Read the model definition and answer for the solid it produces. Units are mm, in the model's axes. A direction names the side the tool comes from. Coordinates: 2 decimals unless noted, no trailing zeros. Order: outer loops, then holes, each group sorted by start corner. A loop starts at its lowest first (then second) coordinate and runs counter-clockwise, first axis right, second up.
```python
from build123d import *

# Parameters (mm, degrees)
F1_DEPTH = 100
F2_R     = 8.25
F3_DEPTH = 130.001
F4_R     = 20


with BuildPart() as f1:
    # F0 (on Top) → F1 (new body, symmetric)
    with BuildSketch(Plane.XY):
        with BuildLine():
            Line((-45, -45), (45, -45))
            ThreePointArc((45, -45), (59.142136, -39.142136), (65, -25))
            Line((65, -25), (65, 45))
            Line((65, 45), (55, 45))
            Line((55, 45), (55, -25))
            ThreePointArc((55, -25), (52.071068, -32.071068), (45, -35))
            Line((45, -35), (-45, -35))
            ThreePointArc((-45, -35), (-52.071068, -32.071068), (-55, -25))
            Line((-55, -25), (-55, 45))
            Line((-55, 45), (-65, 45))
            Line((-65, 45), (-65, -25))
            ThreePointArc((-65, -25), (-59.142136, -39.142136), (-45, -45))
        make_face()
    extrude(amount=F1_DEPTH, both=True)

    # F2 (on face) → F3 (cut, through all)
    with BuildSketch(Plane.YZ.offset(65)):
        with Locations((0, 62.5)):
            Circle(F2_R)
        with Locations((0, -62.5)):
            Circle(F2_R)
    extrude(amount=-F3_DEPTH, mode=Mode.SUBTRACT)

    # F4
    f4_edges = [f1.edges().sort_by_distance(p)[0] for p in [
        (60, 45, 100),
        (-60, 45, 100),
        (-60, 45, -100),
        (60, 45, -100),
    ]]
    fillet(f4_edges, radius=F4_R)


solid = f1.part
```
1) Determine the mould class of faces 1 (the cylindrical face through (58.986, -39.297, 1.4)), 2 (the cylindrical face through (-59.93, -1.07, 70.68)), 3 (the flat face through (65, 10, 1)), 4 (the cylindrical face through (59.93, 38.986, -94.297)) for opening direction Y: pulls with the +Y half, pulls with the -Y half, needs draft (parallel to the pull), parting line crosses it, or undercut.
A:
face 1: pulls with the -Y half
face 2: undercut
face 3: needs draft
face 4: pulls with the +Y half
2) A cutting plane is placed at B-B, the plane y = 0. Determine the outline of the cut face in (x, z).
A:
outline: (-65, -100) - (-55, -100) - (-55, -70.75) - (-65, -70.75) - close; (-65, -54.25) - (-55, -54.25) - (-55, 54.25) - (-65, 54.25) - close; (-65, 70.75) - (-55, 70.75) - (-55, 100) - (-65, 100) - close; (55, -100) - (65, -100) - (65, -70.75) - (55, -70.75) - close; (55, -54.25) - (65, -54.25) - (65, 54.25) - (55, 54.25) - close; (55, 70.75) - (65, 70.75) - (65, 100) - (55, 100) - close
3) Flat-ended cylindrical pins translate along their axes: pin 1 Ø10 at (x, z) = (21, 19.5) entering from +Y; pin 2 Ø15 at (y, z) = (0, 62.5) entering from -X; pin 3 Ø1 at (x, z) = (51, -62) entering from +Y; pin 4 Ø10 at (y, z) = (-32, -6.5) entering from -X. Find the tip coordinate at first contact, or state that the pin passes through.
A:
pin 1: stops at y = -35
pin 2: passes through
pin 3: stops at y = -32.6
pin 4: stops at x = -64.9
4) A cutting plane is placed at C-C, the plane y = -31.5. Determine the outline of the cut face in (x, z).
A:
outline: (-63.91, -100) - (-52.6, -100) - (-52.6, 100) - (-63.91, 100) - close; (52.6, -100) - (63.91, -100) - (63.91, 100) - (52.6, 100) - close
5) Which of the six approach directions +Z, -Z, +X, -X, +Y, -Y give full straight-line access (tool end or side, diameter ignored) to faces 5 (the flat face through (-1, -45, 1)), 6 (the flat face through (55, 10, 1))?
A:
face 5: +Z, -Z, +X, -X, -Y
face 6: +Z, -Z, +Y
6) Straight lines are drawn through the part: line 1 (Z direction, x = -61, y = 0); line 2 (X direction, y = 40.5, z = 29.5); line 3 (Y direction, x = -21, z = -39). For each, find the intervals that lie inside material, in ascending order.
A:
line 1: z = -100 to -70.75, -54.25 to 54.25, 70.75 to 100
line 2: x = -65 to -55, 55 to 65
line 3: y = -45 to -35
7) A cutting plane is placed at D-D, the plane z = 34. Determine the outline of the cut face in (x, y).
A:
outline: (-65, -25) arc R20 ccw to (-45, -45) - (45, -45) arc R20 ccw to (65, -25) - (65, 45) - (55, 45) - (55, -25) arc R10 cw to (45, -35) - (-45, -35) arc R10 cw to (-55, -25) - (-55, 45) - (-65, 45) - close
8) A cutting plane is placed at A-A, the plane z = 62.5. Determine the outline of the cut face in (x, y), and give its area (3 significant figures).
A:
outline: (-65, -25) arc R20 ccw to (-45, -45) - (45, -45) arc R20 ccw to (65, -25) - (65, -8.25) - (55, -8.25) - (55, -25) arc R10 cw to (45, -35) - (-45, -35) arc R10 cw to (-55, -25) - (-55, -8.25) - (-65, -8.25) - close; (-65, 8.25) - (-55, 8.25) - (-55, 45) - (-65, 45) - close; (55, 8.25) - (65, 8.25) - (65, 45) - (55, 45) - close
area: 2,440 mm2
